Model file for the job. Use its own axes, mm. A direction names the side the tool comes from. Coordinates: 2 decimals unless noted, no trailing zeros. Write each loop counter-clockwise with the first axis right and the second up, starting at its lowest first coordinate (ties: lowest second). Pieces come first, ordered by that corner, then holes. Notation, with made-up numbers: (19, 27) -> (64, 27) arc R13 ccw to (64, 40) -> close; hole circle Ø2 at (87.25, 71.25). An arc over 180 degrees is marked (long way). Write item = value, one per line. Start each with the question number.
from build123d import *

# Parameters (mm, degrees)
SKETCH1_W                      = 120
SKETCH1_H                      = 42.5
BOSS_EXTRUDE1_DEPTH            = 7
SKETCH2_R                      = 19.1
CUT_EXTRUDE1_DEPTH             = 3
SKETCH3_R                      = 15
CUT_EXTRUDE2_DEPTH             = 65.595375221
M5X0_8_TAPPED_HOLE3_D          = 4.2
M5X0_8_TAPPED_HOLE3_DEPTH      = 14
M5X0_8_TAPPED_HOLE3_TIP        = 1.2618073
SKETCH5_R                      = 6
CUT_EXTRUDE4_DEPTH             = 66.173326599
M5X0_8_TAPPED_HOLE2_AT_2_COUNT = 2
M5X0_8_TAPPED_HOLE2_AT_2_PITCH = 28
SKETCH6_R                      = 1.25
CUT_EXTRUDE5_DEPTH             = 10
M5X0_8_TAPPED_HOLE1_REACH      = 75.86
M5X0_8_TAPPED_HOLE1_BORE_R     = 2.1
SKETCH16_W                     = 14
SKETCH16_H                     = 42.5
BOSS_EXTRUDE2_DEPTH            = 11
SKETCH17_W                     = 11
SKETCH17_H                     = 30
CUT_EXTRUDE6_DEPTH             = 7
M3X0_5_TAPPED_HOLE1_D          = 2.5
SKETCH21_W                     = 10
SKETCH21_H                     = 14
CUT_EXTRUDE7_DEPTH             = 75.441671835
FILLET1_R                      = 3
CHAMFER1_SIZE                  = 0.5


with BuildPart() as part:
    # Sketch1 → Boss-Extrude1 (new, symmetric)
    with BuildSketch(Plane.XY):
        Rectangle(SKETCH1_W, SKETCH1_H)
    extrude(amount=BOSS_EXTRUDE1_DEPTH, both=True)

    # Sketch2 → Cut-Extrude1 (cut)
    with BuildSketch(Plane.XY.offset(7)):
        Circle(SKETCH2_R)
    extrude(amount=-CUT_EXTRUDE1_DEPTH, mode=Mode.SUBTRACT)

    # Sketch3 → Cut-Extrude2 (cut, through all)
    with BuildSketch(Plane.XY.offset(4)):
        Circle(SKETCH3_R)
    extrude(amount=-CUT_EXTRUDE2_DEPTH, mode=Mode.SUBTRACT)

    # M5x0.8 Tapped Hole3
    with Locations(Plane.XY.offset(7)):
        with Locations((-30.248022392, -14.104884486), (30.248022392, 14.104884486)):
            Hole(M5X0_8_TAPPED_HOLE3_D / 2, depth=M5X0_8_TAPPED_HOLE3_DEPTH)
            with Locations((0, 0, -(M5X0_8_TAPPED_HOLE3_DEPTH + M5X0_8_TAPPED_HOLE3_TIP / 2))):  # 118° drill point
                Cone(0, M5X0_8_TAPPED_HOLE3_D / 2, M5X0_8_TAPPED_HOLE3_TIP, mode=Mode.SUBTRACT)

    # Sketch5 → Cut-Extrude4 (cut, through all)
    with BuildSketch(Plane.XY.offset(7)):
        with Locations((-50, 3.4)):
            Circle(SKETCH5_R)
        with Locations((50, 3.4)):
            Circle(SKETCH5_R)
    extrude(amount=-CUT_EXTRUDE4_DEPTH, mode=Mode.SUBTRACT)

    # Sketch10 → M5x0.8 Tapped Hole2 (revolve, cut)
    with BuildSketch(Plane(origin=(-50, -21.25, 0), x_dir=(0, 0, -1), z_dir=(1, 0, 0))):
        Polygon((0, 0), (0, 15.2618073), (2.1, 14), (2.1, 0), align=None)
    m5x0_8_tapped_hole2 = revolve(axis=Axis((-50, -27.6, 0), (0, 1, 0)), mode=Mode.SUBTRACT)

    # M5x0.8 Tapped Hole2 at 2: M5x0.8 Tapped Hole2 ×2
    with Locations(*[(i * M5X0_8_TAPPED_HOLE2_AT_2_PITCH, 0, 0) for i in range(1, M5X0_8_TAPPED_HOLE2_AT_2_COUNT)]):
        add(m5x0_8_tapped_hole2, mode=Mode.SUBTRACT)

    # Sketch6 → Cut-Extrude5 (cut)
    with BuildSketch(Plane.XZ.offset(21.25)):
        with Locations(Location((-36, 0, 0), (0, 0, 270))):
            Circle(SKETCH6_R)
    cut_extrude5 = extrude(amount=-CUT_EXTRUDE5_DEPTH, mode=Mode.SUBTRACT)

    # Mirror1: M5x0.8 Tapped Hole2, Cut-Extrude5 across plane
    add(m5x0_8_tapped_hole2.mirror(Plane(origin=(0, 0, 0), x_dir=(0, 0, 1), z_dir=(1, 0, 0))), mode=Mode.SUBTRACT)
    add(cut_extrude5.mirror(Plane(origin=(0, 0, 0), x_dir=(0, 0, 1), z_dir=(1, 0, 0))), mode=Mode.SUBTRACT)

    # Mirror1 copy 1 sketch → Mirror1 copy 1 (revolve, cut)
    with BuildSketch(Plane(origin=(22, -21.25, 0), x_dir=(0, 0, -1), z_dir=(-1, 0, 0))):
        Polygon((0, 0), (0, -15.2618073), (2.1, -14), (2.1, 0), align=None)
    revolve(axis=Axis((22, -27.6, 0), (0, -1, 0)), mode=Mode.SUBTRACT)

    # M5x0.8 Tapped Hole1 bore → M5x0.8 Tapped Hole1 (cut, up to next)
    with BuildSketch(Plane(origin=(0, 21.25, 0), x_dir=(1, 0, 0), z_dir=(0, 1, 0)), mode=Mode.PRIVATE) as m5x0_8_tapped_hole1_sk1:
        with Locations((-50, 0)):
            Circle(M5X0_8_TAPPED_HOLE1_BORE_R)
    m5x0_8_tapped_hole1_tool1 = extrude(m5x0_8_tapped_hole1_sk1.sketch, amount=-M5X0_8_TAPPED_HOLE1_REACH, mode=Mode.PRIVATE) & part.part
    # M5x0.8 Tapped Hole1 bore → M5x0.8 Tapped Hole1 (cut, up to next)
    with BuildSketch(Plane(origin=(0, 21.25, 0), x_dir=(1, 0, 0), z_dir=(0, 1, 0)), mode=Mode.PRIVATE) as m5x0_8_tapped_hole1_sk2:
        with Locations((50, 0)):
            Circle(M5X0_8_TAPPED_HOLE1_BORE_R)
    m5x0_8_tapped_hole1_tool2 = extrude(m5x0_8_tapped_hole1_sk2.sketch, amount=-M5X0_8_TAPPED_HOLE1_REACH, mode=Mode.PRIVATE) & part.part
    add(m5x0_8_tapped_hole1_tool1.solids().sort_by_distance((-50, 21.25, 0))[0], mode=Mode.SUBTRACT)
    add(m5x0_8_tapped_hole1_tool2.solids().sort_by_distance((50, 21.25, 0))[0], mode=Mode.SUBTRACT)

    # Sketch16 → Boss-Extrude2 (add)
    with BuildSketch(Plane.ZY.offset(60)):
        Rectangle(SKETCH16_W, SKETCH16_H)
    extrude(amount=BOSS_EXTRUDE2_DEPTH)

    # Sketch17 → Cut-Extrude6 (cut)
    with BuildSketch(Plane.XY.offset(7)):
        with Locations((-65.5, 2)):
            Rectangle(SKETCH17_W, SKETCH17_H)
    extrude(amount=-CUT_EXTRUDE6_DEPTH, mode=Mode.SUBTRACT)

    # M3x0.5 Tapped Hole1 (through all)
    with Locations(Plane.XY):
        with Locations((-65.5, 12), (-65.5, -8)):
            Hole(M3X0_5_TAPPED_HOLE1_D / 2)

    # Sketch21 → Cut-Extrude7 (cut, through all)
    with BuildSketch(Plane.XY):
        with Locations((-66, 2)):
            Rectangle(SKETCH21_W, SKETCH21_H)
    extrude(amount=-CUT_EXTRUDE7_DEPTH, mode=Mode.SUBTRACT)

    # Fillet1
    fillet1_edges = [part.edges().sort_by_distance(p)[0] for p in [
        (-61, 9, -3.5),
        (-61, -5, -3.5),
        (-60, 17, 3.5),
        (-60, -13, 3.5),
    ]]
    fillet(fillet1_edges, radius=FILLET1_R)

    # Chamfer1
    chamfer1_edges = [part.edges().sort_by_distance(p)[0] for p in [
        (-71, -9, 0),
        (-71, -13.125, -7),
        (-71, -5, -3.5),
        (-71, 9, -3.5),
        (-67.5, -5, -7),
        (-67.5, -5, 0),
        (-5.5, -21.25, 7),
        (-61, 2, 0),
        (-61, 2, -7),
        (-67.5, 9, 0),
        (-67.5, 9, -7),
        (-60, 2, 7),
        (-67, 17, 7),
        (-61.878679656, -4.121320344, 0),
        (-61.878679656, -4.121320344, -7),
        (-61.878679656, 8.121320344, 0),
        (-61.878679656, 8.121320344, -7),
        (-60.878679656, -12.121320344, 7),
        (-19.1, 0, 7),
        (-60.878679656, 16.121320344, 7),
        (-15, 0, -7),
        (-15, 0, 4),
        (-56, 3.4, -7),
        (-56, 3.4, 7),
        (44, 3.4, -7),
        (44, 3.4, 7),
        (60, 0, 7),
        (-5.5, -21.25, -7),
        (-36, -21.25, 1.25),
        (-5.5, 21.25, -7),
        (60, 0, -7),
        (36, -21.25, 1.25),
        (-5.5, 21.25, 7),
        (60, -21.25, 0),
        (60, 21.25, 0),
        (-71, -17.125, 7),
        (-71, 21.25, 0),
        (-71, 15.125, -7),
        (-71, -21.25, 0),
        (-71, 19.125, 7),
        (-71, 13, 0),
        (-71, -13, 3.5),
        (-71, 17, 3.5),
        (-67, -13, 7),
    ]]
    chamfer(chamfer1_edges, length=CHAMFER1_SIZE)


solid = part.part
(1) Saw through at C-C (z = 5.25). Give the cut face in (x, y), then the cut area to 3 significant figures.
(2) Drill centre lines: line 1 along Z through (x, y) = (-50, 13); line 2 along X through (y, z) = (-2, 4.25) (3 decimals); line 3 along X through (y, z) = (16, -6). Where is each one in solid material? Low to high.
(3) Drop flat-ended pins along their axis: pin 1 Ø0.8 at (x, z) = (-35.5, 0.5) entering from -Y; pin 2 Ø2.5 at (x, z) = (-22, 0) entering from -Y; pin 3 Ø5 at (y, z) = (3.5, -4) entering from -X. Give the stop position or say it passes through.
(4) Saw through at A-A (x = 0). Give the cut face in (y, z), then the cut area to 3 significant figures.
(5) Saw through at B-B (x = 36). Give the cut face in (y, z).
(6) 3-axis set-ups, long thin cutter, end or side, ignore diameter. For faces 1 (the face through (-60.9, 16.14, 3.2)), 2 (the face through (-61.86, -4.1, -3.54)), 3 (the face through (-48.06, 15.22, 0.8)), 4 (the face through (47.95, -14.35, 0.46)), 5 (the face through (-61.759, -4.193, -6.635)): which of +Z, -Z, +X, -X, +Y, -Y reach the whole face in a straight line?
(7) Mould opens along Y. For faces 6 (the face through (-22.31, -6.21, -0.2)), 7 (the face through (-60.9, -12.14, 3.2)), 8 (the face through (-19, 0, -7)) say: released by +Y, released by -Y, zero draft, split by the parting line, or undercut.
Returned:
q1.outline = (-71, -20.75) -> (-70.5, -21.25) -> (59.5, -21.25) -> (60, -20.75) -> (60, 20.75) -> (59.5, 21.25) -> (-70.5, 21.25) -> (-71, 20.75) -> (-71, 17.5) -> (-70.5, 17) -> (-63, 17) arc R3 cw to (-60, 14) -> (-60, -10) arc R3 cw to (-63, -13) -> (-70.5, -13) -> (-71, -13.5) -> close; hole circle Ø12 at (-50, 3.4); hole circle Ø4.2 at (-30.25, -14.1); hole circle Ø38.2 at (0, 0); hole circle Ø4.2 at (30.25, 14.1); hole circle Ø12 at (50, 3.4)
q1.area = 3,840 mm2
q2.line_1 = -7 to -2.1, 2.1 to 7
q2.line_2 = -60 to -52.615, -47.385 to -18.995, 18.995 to 47.385, 52.615 to 60
q2.line_3 = -71 to 29.34, 31.15 to 60
q3.pin_1 = -11.25
q3.pin_2 = -6.74
q3.pin_3 = -61
q4.outline = (-21.25, -6.5) -> (-20.75, -7) -> (-15.5, -7) -> (-15, -6.5) -> (-15, 3.5) -> (-15.5, 4) -> (-19.1, 4) -> (-19.1, 6.5) -> (-19.6, 7) -> (-20.75, 7) -> (-21.25, 6.5) -> close; (15, -6.5) -> (15.5, -7) -> (20.75, -7) -> (21.25, -6.5) -> (21.25, 6.5) -> (20.75, 7) -> (19.6, 7) -> (19.1, 6.5) -> (19.1, 4) -> (15.5, 4) -> (15, 3.5) -> close
q4.area = 149 mm2
q5.outline = (-21.25, -6.5) -> (-20.75, -7) -> (20.75, -7) -> (21.25, -6.5) -> (21.25, 6.5) -> (20.75, 7) -> (-20.75, 7) -> (-21.25, 6.5) -> (-21.25, 1.75) -> (-20.75, 1.25) -> (-11.25, 1.25) -> (-11.25, -1.25) -> (-20.75, -1.25) -> (-21.25, -1.75) -> close
q6.face_1 = +Z, -X
q6.face_2 = +Z, -Z, -X
q6.face_3 = +Y
q6.face_4 = -Y
q6.face_5 = -Z, -X
q7.face_6 = released by -Y
q7.face_7 = undercut
q7.face_8 = zero draft
